Geometry: final body of the model. Coordinates: model frame, mm. A direction names the side the tool comes from. Round coordinates to 2 decimals unless told otherwise and drop trailing zeros. Order: outer loops, then holes, each group sorted by start corner. A loop starts at its lowest first (then second) coordinate and runs counter-clockwise, first axis right, second up. Notation, with made-up numbers: M 78.5,-37.75 L 116.5,-37.75 A22 ccw 116.5,-2.75 Z; hole C 72.5,65 d10. An arc over 180 degrees is marked long. Return JSON: item names as keys, results as strings. Group by question number.
Q1. Access query for faces 1 (the face through (2.38, -10.74, 2.74)), 2 (the face through (2, 8, 2)). Directions: +Z, -Z, +X, -X, +Y, -Y. A direction counts if a zero-diameter tool reaches every point of the face in a straight line with its end or side. Return the directions, or none.
Q2. Cut plane C-C on z = 1.5. Output: boundary loops of the cut face in (x, y).
Q3. Cut plane A-A on y = 0. Output: boundary loops of the cut face in (x, z).
Q4. Mould query, pull axis Z, two halves, no side actions, for faces 3 (the face through (1.73, 7.81, 0.03)), 4 (the face through (-7, 0, 4.5)), 5 (the face through (-7, 0, -4.5)), 6 (the face through (2.38, 10.74, -2.74)). Classes: released by +Z, released by -Z, zero draft, split by the parting line, or undercut.
Q5. Ray query, probe 1 along Y at (x, z) = (0, 0); probe 2 along X at (y, z) = (0, 2.25); probe 3 along Z at (x, y) = (8.25, -5.75). Return the intervals inside material, ascending.
Q6. Cut plane D-D on z = 2.75. Output: boundary loops of the cut face in (x, y).
Q7. Contact query for flat-ended pins moving along their axis: pin 1 (5 mm diameter, centred on x = 8.5, z = 3.5, fed in from +Y); pin 2 (1.5 mm diameter, centred on y = 1, z = -3, fed in from -X); pin 3 (2 mm diameter, centred on x = 5.5, z = -0.5, fed in from +Y). Output: stop coordinate, or through.
Autodesk Inventor part; units mm, degrees
ref_plane "YZ Plane" through (0, 0, 0) normal (1, 0, 0) x (0, 1, 0)
ref_plane "XZ Plane" through (0, 0, 0) normal (0, 1, 0) x (-1, 0, 0)
ref_plane "XY Plane" through (0, 0, 0) normal (0, 0, 1) x (1, 0, 0)
sketch "Sketch1" plane through (0, 0, 0) normal (0, 1, 0) x (-1, 0, 0)
  line L0 (0, 0) -> (6, 0) construction
  line L1 (6, 0) -> (11, 0) construction
  line L2 (6, 0) -> (6, -4.5)
  line L3 (6, -4.5) -> (10, -4.5)
  line L4 (11, -3.5) -> (11, -2)
  line L5 (11, -2) -> (8, -2)
  line L6 (8, -2) -> (8, 0)
  arc A0 (10, -4.5) -> (11, -3.5) centre (10, -3.5) ccw
  line L7 (6, 0) -> (6, 4.5)
  line L8 (6, 4.5) -> (10, 4.5)
  line L9 (11, 3.5) -> (11, 2)
  line L10 (11, 2) -> (8, 2)
  line L11 (8, 2) -> (8, 0)
  arc A1 (11, 3.5) -> (10, 4.5) centre (10, 3.5) ccw
  line L12 (0, -6.5899) -> (0, 6.5899)
  point P0 (11, -4.5)
  point P1 (11, 4.5)
  dimension "d0" = 6
  dimension "d1" = 5
  dimension "d2" = 4.5
  dimension "d3" = 5
  dimension "d4" = 2.5
  dimension "d5" = 3
  dimension "d6" = 1
revolve "Revolution1" add sketch "Sketch1" angle 360 about axis through (0, 0, -10) along (0, 0, 1)
properties part number "Tarot_12mm_Rubber" material "Rubber"
Result sheet:
{
 "1": {"face 1": "+Z, -Z", "face 2": "none"},
 "2": {"outline": "C 0,0 d16; hole C 0,0 d12"},
 "3": {"outline": "M -11,-3.5 A1 ccw -10,-4.5 L -6,-4.5 L -6,4.5 L -10,4.5 A1 ccw -11,3.5 L -11,2 L -8,2 L -8,-2 L -11,-2 Z; M 6,-4.5 L 10,-4.5 A1 ccw 11,-3.5 L 11,-2 L 8,-2 L 8,2 L 11,2 L 11,3.5 A1 ccw 10,4.5 L 6,4.5 Z"},
 "4": {"face 3": "undercut", "face 4": "released by +Z", "face 5": "released by -Z", "face 6": "zero draft"},
 "5": {"probe 1": "y = -8 to -6, 6 to 8", "probe 2": "x = -11 to -6, 6 to 11", "probe 3": "z = -4.5 to -2, 2 to 4.5"},
 "6": {"outline": "C 0,0 d22; hole C 0,0 d12"},
 "7": {"pin 1": "stops at y = 9.22", "pin 2": "stops at x = -11", "pin 3": "stops at y = 6.61"}
}
